```python
from build123d import *

# Parameters (mm, degrees)
SKETCH2_W               = 60
SKETCH2_H               = 60
BOSS_EXTRUDE1_DEPTH     = 150
SKETCH3_W               = 20
SKETCH3_H               = 60
BOSS_EXTRUDE2_DEPTH     = 30
BOSS_EXTRUDE3_DEPTH     = 20
BOSS_EXTRUDE4_START     = -20
BOSS_EXTRUDE4_DEPTH     = 20
SKETCH6_W               = 60
SKETCH6_H               = 20
BOSS_EXTRUDE5_DEPTH     = 30
BOSS_EXTRUDE6_DEPTH     = 20
CUT_EXTRUDE2_DEPTH      = 5
CUT_EXTRUDE2_DEPTH_BACK = 130
CUT_EXTRUDE2_START      = -10
SKETCH8_W               = 50.5
SKETCH8_H               = 50.5
SKETCH9_R               = 4.15
CUT_EXTRUDE3_DEPTH      = 130
SKETCH11_R              = 4.15
CUT_EXTRUDE4_DEPTH      = 212.144400343
SKETCH12_R              = 4.15
CUT_EXTRUDE5_DEPTH      = 212.144400343


with BuildPart() as part:
    # Sketch2 → Boss-Extrude1 (new body)
    with BuildSketch(Plane.XY):
        Rectangle(SKETCH2_W, SKETCH2_H)
    extrude(amount=BOSS_EXTRUDE1_DEPTH)

    # Sketch3 → Boss-Extrude2 (add)
    with BuildSketch(Plane(origin=(0, 0, 0), x_dir=(-1, 0, 0), z_dir=(0, 0, -1))):
        with Locations((20, 0)):
            Rectangle(SKETCH3_W, SKETCH3_H)
        with Locations((-20, 0)):
            Rectangle(SKETCH3_W, SKETCH3_H)
    extrude(amount=BOSS_EXTRUDE2_DEPTH)

    # Sketch4 → Boss-Extrude3 (add)
    with BuildSketch(Plane(origin=(30, 0, 0), x_dir=(0, 0, -1), z_dir=(1, 0, 0))):
        with BuildLine():
            Line((30, 30), (30, -30))
            ThreePointArc((30, -30), (55.138874415, 0), (30, 30))
        make_face()
    extrude(amount=-BOSS_EXTRUDE3_DEPTH)

    # Sketch5 → Boss-Extrude4 (add)
    with BuildSketch(Plane.ZY.offset(30).offset(BOSS_EXTRUDE4_START)):
        with BuildLine():
            Line((-30, -30), (-30, 30))
            ThreePointArc((-30, 30), (-55.138874415, 0), (-30, -30))
        make_face()
    extrude(amount=BOSS_EXTRUDE4_DEPTH)

    # Sketch6 → Boss-Extrude5 (add)
    with BuildSketch(Plane.XY.offset(150)):
        Rectangle(SKETCH6_W, SKETCH6_H)
    extrude(amount=BOSS_EXTRUDE5_DEPTH)

    # Sketch7 → Boss-Extrude6 (add)
    with BuildSketch(Plane(origin=(0, 10, 0), x_dir=(1, 0, 0), z_dir=(0, 1, 0))):
        with BuildLine():
            Line((30, -180), (-30, -180))
            ThreePointArc((-30, -180), (0, -205.138874415), (30, -180))
        make_face()
    extrude(amount=-BOSS_EXTRUDE6_DEPTH)

    # Sketch8 → Cut-Extrude2 (cut, two sides: drawn at the far end of the back side and taken through both)
    with BuildSketch(Plane.XY.offset(150).offset(CUT_EXTRUDE2_START - CUT_EXTRUDE2_DEPTH_BACK)):
        Rectangle(SKETCH8_W, SKETCH8_H)
    extrude(amount=CUT_EXTRUDE2_DEPTH + CUT_EXTRUDE2_DEPTH_BACK, mode=Mode.SUBTRACT)

    # Sketch9 → Cut-Extrude3 (cut)
    with BuildSketch(Plane(origin=(0, -10, 0), x_dir=(-1, 0, 0), z_dir=(0, -1, 0))):
        with Locations(Location((0, -180, 0), (0, 0, 90))):
            Circle(SKETCH9_R)
    extrude(amount=-CUT_EXTRUDE3_DEPTH, mode=Mode.SUBTRACT)

    # Sketch11 → Cut-Extrude4 (cut, through all)
    with BuildSketch(Plane.ZY.offset(-10)):
        with Locations(Location((-30, 0, 0), (0, 0, 270))):
            Circle(SKETCH11_R)
    extrude(amount=-CUT_EXTRUDE4_DEPTH, mode=Mode.SUBTRACT)

    # Sketch12 → Cut-Extrude5 (cut, through all)
    with BuildSketch(Plane(origin=(-10, 0, 0), x_dir=(0, 0, -1), z_dir=(1, 0, 0))):
        with Locations(Location((30, 0, 0), (0, 0, 270))):
            Circle(SKETCH12_R)
    extrude(amount=-CUT_EXTRUDE5_DEPTH, mode=Mode.SUBTRACT)


solid = part.part
```
Geometry: final body of the model. Coordinates: model frame, mm. A direction names the side the tool comes from. Round coordinates to 2 decimals unless told otherwise and drop trailing zeros. Write each loop counter-clockwise with the first axis right and the second up, starting at its lowest first coordinate (ties: lowest second). Pieces come first, ordered by that corner, then holes.
Item 1: Material intervals for L1, parallel to Z at x = -0.5, y = -4.5; L2, parallel to X at y = -15, z = 116; L3, parallel to Z at x = 3, y = -8.5, sorted ascending.
Item 2: Section query A-A (y = 0). Return loops of the section in (x, z), plus the area to 3 significant figures.
Item 3: Section query B-B (x = 0). Return loops of the section in (y, z).
Item 4: Pin query (flat end, axial travel): P1, Ø12, axis at x = 6.5, y = -7, coming from the -Z side; P2, Ø22, axis at x = 9.5, y = 25, coming from the +Z side; P3, Ø7.5, axis at y = 0, z = -30, coming from the -X side; P4, Ø16.5, axis at x = 4, z = 187, coming from the +Y side. Return the tip coordinate at first contact, or that it passes through.
Item 5: Set-up query: faces 4 (the face through (10, 0, -21)), 5 (the face through (0, 25.25, 77)), 6 (the face through (20.14, -0.595, -55.133)), 7 (the face through (30, 0, 64)), 8 (the face through (0, 10, 171)). Return all of +Z, -Z, +X, -X, +Y, -Y with unobstructed straight access to the full face (end or side cutting, diameter ignored); none if empty.
Item 6: Section query C-C (z = 85). Return loops of the section in (x, y).
Item 7: Mould query, pull axis Z, two halves, no side actions, for faces 1 (the face through (0, -20, 150)), 2 (the face through (0, -30, 61)), 3 (the face through (0, -25.25, 77)). Classes: +Z half, -Z half, draft (parallel to the pull), parting line (faces both ways), or undercut.
Item 8: Section query D-D (x = 21). Return loops of the section in (y, z).
Completed:
1. L1: z = 0 to 10, 145 to 175.88, 184.12 to 205.13
1. L2: x = -30 to -25.25, 25.25 to 30
1. L3: z = 0 to 10, 145 to 177.13, 182.87 to 204.99
2. outline: (-30, -55.14) - (-10, -55.14) - (-10, -34.15) - (-30, -34.15) - close; (-30, -25.85) - (-10, -25.85) - (-10, 0) - (10, 0) - (10, -25.85) - (30, -25.85) - (30, 180) arc R30.47 ccw to (-30, 180) - close; (10, -55.14) - (30, -55.14) - (30, -34.15) - (10, -34.15) - close; hole (-25.25, 10) - (25.25, 10) - (25.25, 145) - (-25.25, 145) - close; hole circle Ø8.3 at (0, 180)
2. area: 6,940 mm2
3. outline: (-30, 0) - (30, 0) - (30, 150) - (10, 150) - (10, 175.85) - (-10, 175.85) - (-10, 150) - (-30, 150) - close; (-10, 184.15) - (10, 184.15) - (10, 205.14) - (-10, 205.14) - close; hole (-25.25, 10) - (25.25, 10) - (25.25, 145) - (-25.25, 145) - close
4. P1: stops at z = -55.06
4. P2: stops at z = 150
4. P3: passes through
4. P4: stops at y = 10
5. face 4: -Z, +Y, -Y
5. face 5: none
5. face 6: -Z, +X, -X
5. face 7: +Z, -Z, +X, +Y, -Y
5. face 8: +Z, +X, -X, +Y
6. outline: (-30, -30) - (30, -30) - (30, 30) - (-30, 30) - close; hole (-25.25, -25.25) - (25.25, -25.25) - (25.25, 25.25) - (-25.25, 25.25) - close
7. face 1: +Z half
7. face 2: draft
7. face 3: undercut
8. outline: (-30, -30) arc R30.47 ccw to (30, -30) - (30, 150) - (10, 150) - (10, 196.75) - (-10, 196.75) - (-10, 150) - (-30, 150) - close; hole (-25.25, 10) - (25.25, 10) - (25.25, 145) - (-25.25, 145) - close; hole circle Ø8.3 at (0, -30)
